from build123d import *

# Parameters (mm, degrees)
SKETCH3_W                = 0.428843097
SKETCH3_H                = 18.90052945
CUT_EXTRUDE1_DEPTH       = 14.99883388
CIRPATTERN1_COUNT        = 6
BOSS_EXTRUDE1_DEPTH      = 27.94
BOSS_EXTRUDE1_DEPTH_BACK = 27.94
SKETCH5_R                = 2.237093308


with BuildPart() as part:
    # Sketch1 → Revolve1 (revolve)
    with BuildSketch(Plane.XY, mode=Mode.PRIVATE) as revolve1_sk:
        Polygon((2.237093308, -12.065), (3.175, -6.35), (3.175, 6.35), (2.237093308, 12.065), align=None)
    revolve(revolve1_sk.sketch.rotate(Axis((0, 6.041374164, 0), (0, -1, 0)), 90), axis=Axis((0, 6.041374164, 0), (0, -1, 0)))

    # Sketch3 → Cut-Extrude1 (cut, through all)
    with BuildSketch(Plane.XY.offset(3.175)):
        with Locations((-3.029889302, -0.659045193)):
            Rectangle(SKETCH3_W, SKETCH3_H)
    cut_extrude1 = extrude(amount=-CUT_EXTRUDE1_DEPTH, mode=Mode.SUBTRACT)

    # CirPattern1: Cut-Extrude1 ×6 about axis
    cirpattern1_axis = Axis((0, 0, 0), (0, 1, 0))
    for i in range(1, CIRPATTERN1_COUNT):
        add(cut_extrude1.rotate(cirpattern1_axis, i * 360 / CIRPATTERN1_COUNT), mode=Mode.SUBTRACT)

    # Sketch5 → Boss-Extrude1 (add, two sides: drawn at the far end of the back side and taken through both)
    with BuildSketch(Plane(origin=(0, 0, 0), x_dir=(1, 0, 0), z_dir=(0, 1, 0)).offset(-BOSS_EXTRUDE1_DEPTH_BACK)):
        with Locations(Location((0, 0, 0), (0, 0, 270))):
            Circle(SKETCH5_R)
    extrude(amount=BOSS_EXTRUDE1_DEPTH + BOSS_EXTRUDE1_DEPTH_BACK)


solid = part.part
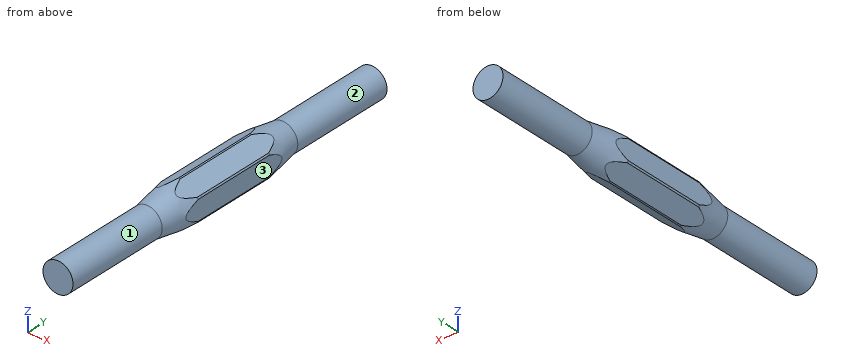
Verification items for the finished model (mm, model axes). Face numbers are marked on the shaded views. A direction names the side the tool comes from. Give positions to 0.01 mm unless a question says otherwise; leave off trailing zeros. Order: outer loops, then holes, each group sorted by start corner. A loop starts at its lowest first (then second) coordinate and runs counter-clockwise, first axis right, second up. Notation, with made-up numbers: M 69.25,65 L 97.25,65 A14 ccw 97.25,73 Z; hole C 46,-19.75 d9. An arc over 180 degrees is marked long. Use one line per item in the form item = value. Start each with the question number.
Q1. Scan lines: line 1 along Z through (x, y) = (0.1, 20); line 2 along Z through (x, y) = (0.1, 10); line 3 along X through (y, z) = (-17, -2). Record each from-to range of solid material in increasing order. Write a range as [from, to].
Q2. Go/stop test with flat-tipped pins: pin 1 Ø1.5 at (y, z) = (-18.5, -0.5) entering from +X; pin 2 Ø3 at (x, y) = (2, 11) entering from -Z. Record where each tip stops, or that it passes through.
Q3. Access from +Z, -Z, +X, -X, +Y, -Y to the whole of each face (thin tool, end or side, straight path). Record for the marked faces 1, 2 and 3.
Q4. Section check B-B (y = 0). Enter the section's corners in (x, z) (3 decimals).
Q5. Section check C-C (y = 14.5). Enter the section's corners in (x, z).
Q6. Section check A-A (z = 0). Enter the section's corners in (x, y) (3 decimals), then the cut area to 3 significant figures.
Evaluation:
q1.line_1 = [-2.23, 2.23]
q1.line_2 = [-2.57, 2.57]
q1.line_3 = [-1, 1]
q2.pin_1 = 2.24
q2.pin_2 = -2.44
q3.face_1 = -Y
q3.face_2 = +Y
q3.face_3 = +Z, -Z, +X, +Y, -Y
q4.outline = M -2.815,-1.468 A3.175 ccw -2.679,-1.704 L -0.137,-3.172 A3.175 ccw 0.137,-3.172 L 2.679,-1.704 A3.175 ccw 2.815,-1.468 L 2.815,1.468 A3.175 ccw 2.679,1.704 L 0.137,3.172 A3.175 ccw -0.137,3.172 L -2.679,1.704 A3.175 ccw -2.815,1.468 Z
q5.outline = C 0,0 d4.47
q6.outline = M -2.815,-8.541 L -2.237,-12.065 L -2.237,-27.94 L 2.237,-27.94 L 2.237,-12.065 L 2.815,-8.541 L 2.815,8.541 L 2.237,12.065 L 2.237,27.94 L -2.237,27.94 L -2.237,12.065 L -2.815,8.541 Z
q6.area = 274 mm2
